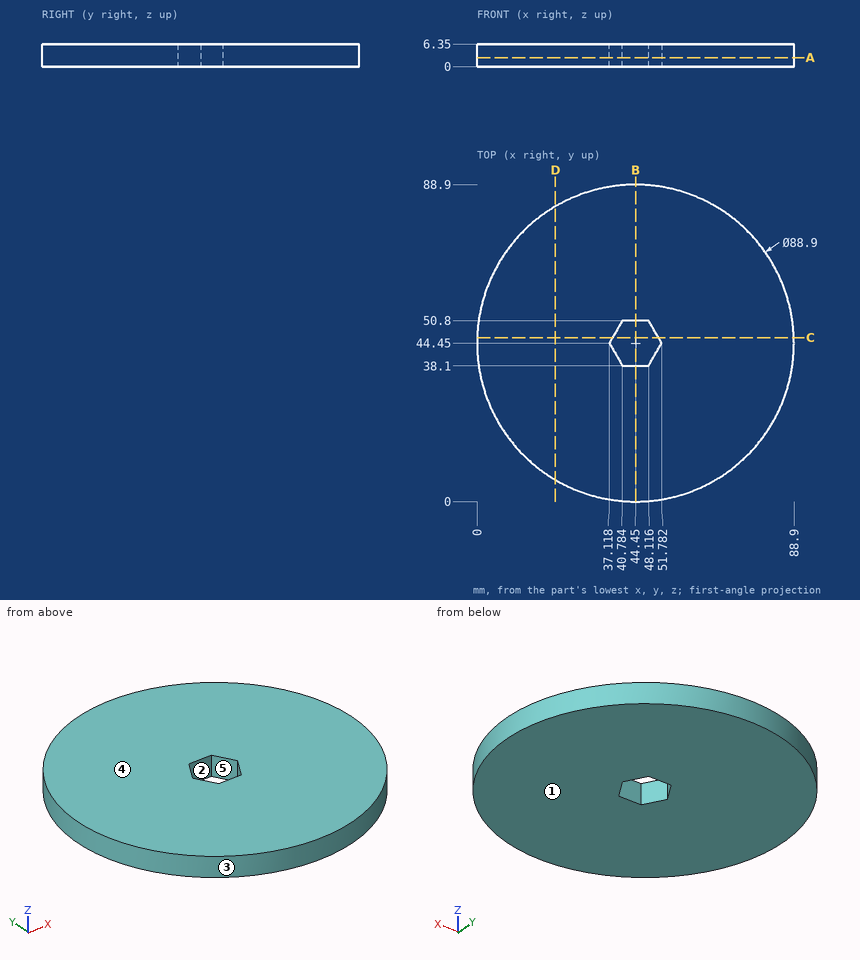
Verification items for this drawing (mm, ordinates from the low corner). A direction names the side the tool comes from. Give positions to 0.01 mm unless a question says otherwise; leave off trailing zeros. Write each loop counter-clockwise with the first axis right and the second up, starting at its lowest first coordinate (ties: lowest second). Pieces come first, ordered by that corner, then holes.
1) Section check D-D, the plane x = 22. Record the boundary of the cut face in (y, z), and give its area (3 significant figures).
2) Section check B-B, the plane x = 44.45. Record the boundary of the cut face in (y, z), and give its area (3 significant figures).
3) Material ranges on L1, parallel to X at y = 49, z = 3.75 (1 decimal); L2, parallel to X at y = 55.5, z = 1 (1 decimal); L3, parallel to Y at x = 60.5, z = 6.25, recorded low to high.
4) Gauge pin test, flat ends, axial feed: pin 1 (1.5 mm diameter, centred on y = 49.5, z = 2.5, fed in from +X); pin 2 (1.9 mm diameter, centred on x = 45, z = 3, fed in from -Y); pin 3 (1.9 mm diameter, centred on x = 42.5, z = 4.5, fed in from +Y). Record the tip position at first contact, or that the pin passes through.
5) Section check A-A, the plane z = 2.5. Record the boundary of the cut face in (x, y), and give its area (3 significant figures).
6) Access from +Z, -Z, +X, -X, +Y, -Y to the whole of each face (thin tool, end or side, straight path). Record for the marked faces 4 and 5.
7) Section check C-C, the plane y = 46. Record the boundary of the cut face in (x, z).
8) Release check for a two-part mould opening along Y. For the marked faces 1, 2 and 3 record: pulls with the +Y half, pulls with the -Y half, needs draft (parallel to the pull), parting line crosses it, or undercut.
Computed:
1. outline: (6.09, 0) - (82.81, 0) - (82.81, 6.35) - (6.09, 6.35) - close
1. area: 487 mm2
2. outline: (0, 0) - (38.1, 0) - (38.1, 6.35) - (0, 6.35) - close; (50.8, 0) - (88.9, 0) - (88.9, 6.35) - (50.8, 6.35) - close
2. area: 484 mm2
3. L1: x = 0.2 to 39.7, 49.2 to 88.7
3. L2: x = 1.4 to 87.5
3. L3: y = 3 to 85.9
4. pin 1: stops at x = 88.69
4. pin 2: stops at y = 0
4. pin 3: stops at y = 88.89
5. outline: circle Ø88.9 at (44.45, 44.45); hole (37.12, 44.45) - (40.78, 38.1) - (48.12, 38.1) - (51.78, 44.45) - (48.12, 50.8) - (40.78, 50.8) - close
5. area: 6,070 mm2
6. face 4: +Z, +X, -X, +Y, -Y
6. face 5: +Z, -Z
7. outline: (0.03, 0) - (38.01, 0) - (38.01, 6.35) - (0.03, 6.35) - close; (50.89, 0) - (88.87, 0) - (88.87, 6.35) - (50.89, 6.35) - close
8. face 1: needs draft
8. face 2: undercut
8. face 3: parting line crosses it
